```python
from build123d import *

# Parameters (mm, degrees)
SKETCH1_W           = 20
SKETCH1_H           = 20
BOSS_EXTRUDE1_DEPTH = 20
SKETCH6_W           = 20
SKETCH6_H           = 20
SKETCH7_W           = 4
SKETCH7_H           = 4
CUT_EXTRUDE2_DEPTH  = 1.5
SCALE1_SCALE        = 2


with BuildPart() as part:
    # Sketch1 → Boss-Extrude1 (new body)
    with BuildSketch(Plane.XY):
        Rectangle(SKETCH1_W, SKETCH1_H)
    extrude(amount=BOSS_EXTRUDE1_DEPTH)

    # Sketch6 → entrada furo section 0
    with BuildSketch(Plane.XY.offset(20), mode=Mode.PRIVATE) as entrada_furo_s0:
        Rectangle(SKETCH6_W, SKETCH6_H)
    loft([entrada_furo_s0.sketch, Vertex(0, 0, 1)], mode=Mode.SUBTRACT)

    # Sketch7 → Cut-Extrude2 (cut)
    with BuildSketch(Plane(origin=(0.412147505, 0, 0.21691974), x_dir=(0.465746433, 0, -0.884918222), z_dir=(0.884918222, 0, 0.465746433))):
        with Locations((-11.620373499, 0)):
            Rectangle(SKETCH7_W, SKETCH7_H)
    cut_extrude2 = extrude(amount=-CUT_EXTRUDE2_DEPTH, mode=Mode.SUBTRACT)

    # Mirror1: Cut-Extrude2 across plane
    add(cut_extrude2.mirror(Plane(origin=(0, 0, 0), x_dir=(0, 0, 1), z_dir=(1, 0, 0))), mode=Mode.SUBTRACT)


with BuildPart() as part_1:
    # Scale1: scaled about (0, 0, 7.5441868)
    add(part.part.scale(SCALE1_SCALE).moved(Location((0, 0, -7.5441868))))


solid = part_1.part
```
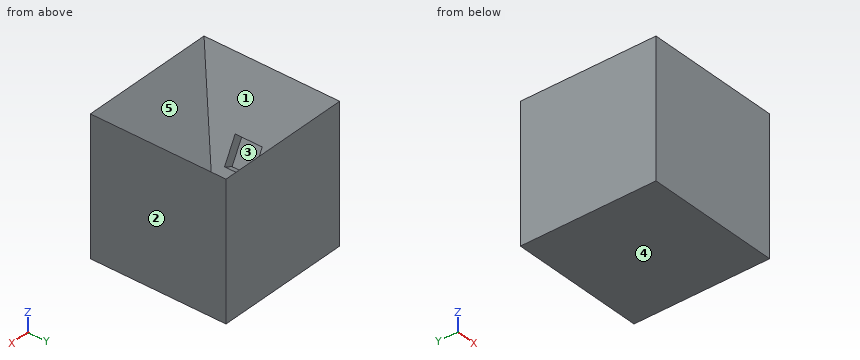
Could you check a few things on this model? Use its own coordinates, in mm. Face numbers are marked on the shaded views. A direction names the side the tool comes from. Round coordinates to 2 decimals unless told otherwise and drop trailing zeros. Loops run counter-clockwise (first coordinate to the right, second up) from the corner with the lowest first, then second, coordinate; pieces in that order, holes last.
Q1. I want a section at A-A (z = 29). Write out the boundary of the cut face in (x, y), and give its area (3 significant figures).
Q2. I want a section at D-D (z = 11). Write out the boundary of the cut face in (x, y), and give its area (3 significant figures).
Q3. On a 3-axis mill with a long thin cutter (end or side, diameter ignored), from which of +Z, -Z, +X, -X, +Y, -Y can I reach the whole of each face in a straight line? I mean the marked faces 1 and 2. Say none if no direction works.
Q4. I want a section at C-C (y = 7.5). Write out the boundary of the cut face in (x, z).
Q5. I want a section at B-B (x = -9). Write out the boundary of the cut face in (y, z).
Q6. Please list where these lines run through material, in increasing order: L1, parallel to Y at x = 10, z = 9; L2, parallel to Y at x = 16, z = 27.5; L3, parallel to X at y = -2.5, z = 30.
Q7. Thinking about a two-plate mould opening in Z: for the marked faces 3, 4 and 5, which applies, pulls with the +Z half, pulls with the -Z half, needs draft (parallel to the pull), parting line crosses it, or undercut?
Answer below:
1. outline: (-20, -20) - (20, -20) - (20, 20) - (-20, 20) - close; hole (-18.18, -18.18) - (18.18, -18.18) - (18.18, 18.18) - (-18.18, 18.18) - close
1. area: 278 mm2
2. outline: (-20, -20) - (20, -20) - (20, 20) - (-20, 20) - close; hole (-12.1, -4) - (-8.71, -4) - (-8.71, -8.71) - (8.71, -8.71) - (8.71, -4) - (12.1, -4) - (12.1, 4) - (8.71, 4) - (8.71, 8.71) - (-8.71, 8.71) - (-8.71, 4) - (-12.1, 4) - close
2. area: 1,240 mm2
3. face 1: +Z
3. face 2: +Z, -Z, +X, +Y, -Y
4. outline: (-20, -7.54) - (20, -7.54) - (20, 32.46) - (7.5, 8.71) - (-7.5, 8.71) - (-20, 32.46) - close
5. outline: (-20, -7.54) - (20, -7.54) - (20, 32.46) - (9, 11.56) - (4, 11.56) - (4, 9.46) - (-4, 9.46) - (-4, 11.56) - (-9, 11.56) - (-20, 32.46) - close
6. L1: y = -20 to -4, 4 to 20
6. L2: y = -20 to -17.39, 17.39 to 20
6. L3: x = -20 to -18.71, 18.71 to 20
7. face 3: undercut
7. face 4: pulls with the -Z half
7. face 5: pulls with the +Z half
